The listing builds one solid part. Answer for the finished solid, in the listing's coordinates (mm). Face numbers are marked on the shaded views. A direction names the side the tool comes from. Round coordinates to 2 decimals unless told otherwise and drop trailing zeros. Write each loop counter-clockwise with the first axis right and the second up, starting at its lowest first coordinate (ties: lowest second). Pieces come first, ordered by that corner, then holes.
(1) A cutting plane is placed at A-A, the plane x = 2.5. Give the vertices of the cut face in (y, z), and give its area (3 significant figures).
(2) A cutting plane is placed at B-B, the plane z = 16. Give the vertices of the cut face in (x, y).
(3) A cutting plane is placed at D-D, the plane z = 5. Give the vertices of the cut face in (x, y), and give its area (3 significant figures).
(4) For the marked faces 1 and 2, determine the directions among +Z, -Z, +X, -X, +Y, -Y from which every point of the face is accessible in a straight line to the end or side of a thin tool.
(5) Each of these flat-tipped pins is pushed along its axis until it touches: pin 1 Ø9 at (y, z) = (4, 10) entering from -X; pin 2 Ø10 at (x, y) = (-7.5, 2.5) entering from +Z. Where does it stop, or does it pass through?
(6) The mould has two halves that part along X. Classify the marked faces 3, 4, 5 and 6: +X half, -X half, draft (parallel to the pull), parting line (faces both ways), or undercut.
(7) Find the intervals of material crossed by probe 1 along X at (y, z) = (10, 6.5); probe 2 along Z at (x, y) = (12, -10.5), in increasing order.
from build123d import *

# Parameters (mm, degrees)
F0_W     = 33.4
F0_H     = 33.4
F0_W_2   = 31
F0_H_2   = 31
F1_DEPTH = 31.7
F2_DEPTH = 1.2
F3_W     = 18
F3_H     = 18
F4_DEPTH = 33.401
F5_W     = 18
F5_H     = 18
F6_DEPTH = 33.401
F7_W     = 18
F7_H     = 18
F8_DEPTH = 31.701


with BuildPart() as f1:
    # F0 (on Top) → F1 (new body)
    with BuildSketch(Plane.XY):
        Rectangle(F0_W, F0_H)
        Rectangle(F0_W_2, F0_H_2, mode=Mode.SUBTRACT)
    extrude(amount=F1_DEPTH)

    # F0 (on Top) → F2 (join)
    with BuildSketch(Plane.XY):
        Rectangle(F0_W_2, F0_H_2)
    extrude(amount=F2_DEPTH)

    # F3 (on face) → F4 (cut, through all)
    with BuildSketch(Plane.XZ.offset(16.7)):
        with Locations((0, 15.85)):
            Rectangle(F3_W, F3_H)
    extrude(amount=-F4_DEPTH, mode=Mode.SUBTRACT)

    # F5 (on face) → F6 (cut, through all)
    with BuildSketch(Plane.YZ.offset(16.7)):
        with Locations((0, 15.85)):
            Rectangle(F5_W, F5_H)
    extrude(amount=-F6_DEPTH, mode=Mode.SUBTRACT)

    # F7 (on face) → F8 (cut, through all)
    with BuildSketch(Plane.XY):
        Rectangle(F7_W, F7_H)
    extrude(amount=F8_DEPTH, mode=Mode.SUBTRACT)


solid = f1.part
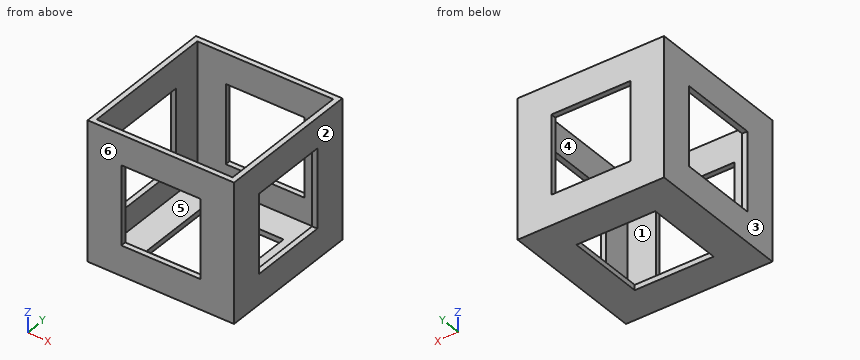
Solutions:
1. outline: (-16.7, 0) - (-9, 0) - (-9, 1.2) - (-15.5, 1.2) - (-15.5, 6.85) - (-16.7, 6.85) - close; (-16.7, 24.85) - (-15.5, 24.85) - (-15.5, 31.7) - (-16.7, 31.7) - close; (9, 0) - (16.7, 0) - (16.7, 6.85) - (15.5, 6.85) - (15.5, 1.2) - (9, 1.2) - close; (15.5, 24.85) - (16.7, 24.85) - (16.7, 31.7) - (15.5, 31.7) - close
1. area: 48.5 mm2
2. outline: (-16.7, -16.7) - (-9, -16.7) - (-9, -15.5) - (-15.5, -15.5) - (-15.5, -9) - (-16.7, -9) - close; (-16.7, 9) - (-15.5, 9) - (-15.5, 15.5) - (-9, 15.5) - (-9, 16.7) - (-16.7, 16.7) - close; (9, -16.7) - (16.7, -16.7) - (16.7, -9) - (15.5, -9) - (15.5, -15.5) - (9, -15.5) - close; (9, 15.5) - (15.5, 15.5) - (15.5, 9) - (16.7, 9) - (16.7, 16.7) - (9, 16.7) - close
3. outline: (-16.7, -16.7) - (16.7, -16.7) - (16.7, 16.7) - (-16.7, 16.7) - close; hole (-15.5, -15.5) - (15.5, -15.5) - (15.5, 15.5) - (-15.5, 15.5) - close
3. area: 155 mm2
4. face 1: +Z
4. face 2: +Z, -Z, +X, +Y, -Y
5. pin 1: stops at x = -16.7
5. pin 2: stops at z = 1.2
6. face 3: -X half
6. face 4: undercut
6. face 5: undercut
6. face 6: draft
7. probe 1: x = -16.7 to -15.5, 15.5 to 16.7
7. probe 2: z = 0 to 1.2
